```python
from build123d import *

# Parameters (mm, degrees)
F1_DEPTH = 254
F2_R     = 15.875
F3_DEPTH = 12.7


# Not quite as in the source:
# - a pattern or mirror of a feature is missing from the dataset's text; its kind, count and spacing are read off the source's solid


with BuildPart() as f1:
    # F0 (on Front) → F1 (new body)
    with BuildSketch(Plane.XZ):
        Polygon((101.6, 116.5001839399), (0, 0), (203.2, 0), align=None)
    extrude(amount=F1_DEPTH)

    # F2 (on face) → F3 (cut)
    with BuildSketch(Plane(origin=(115.4177397592, 0, 100.6559986685), x_dir=(0, 1, 0), z_dir=(0.7536582036, 0, 0.6572665458))):
        with BuildLine():
            Line((-165.875079947, -18.1667619065), (-171.45, -18.1667619065))
            ThreePointArc((-171.45, -18.1667619065), (-209.55, -56.2667619065), (-171.45, -94.3667619065))
            Line((-171.45, -94.3667619065), (-165.875079947, -94.3667619065))
            ThreePointArc((-165.875079947, -94.3667619065), (-127, -88.270559031), (-88.124920053, -94.3667619065))
            Line((-88.124920053, -94.3667619065), (-82.55, -94.3667619065))
            ThreePointArc((-82.55, -94.3667619065), (-44.45, -56.2667619065), (-82.55, -18.1667619065))
            Line((-82.55, -18.1667619065), (-88.124920053, -18.1667619065))
            ThreePointArc((-88.124920053, -18.1667619065), (-127, -24.262964782), (-165.875079947, -18.1667619065))
        make_face()
        with Locations((-171.45, -56.2667619065)):
            Circle(F2_R, mode=Mode.SUBTRACT)
        with Locations((-82.55, -56.2667619065)):
            Circle(F2_R, mode=Mode.SUBTRACT)
    f3 = extrude(amount=-F3_DEPTH, mode=Mode.SUBTRACT)

    # F3_copies: F3 across plane
    add(f3.mirror(Plane(origin=(101.6, 0, 0), x_dir=(0, 0, -1), z_dir=(-1, 0, 0))), mode=Mode.SUBTRACT)


solid = f1.part
```
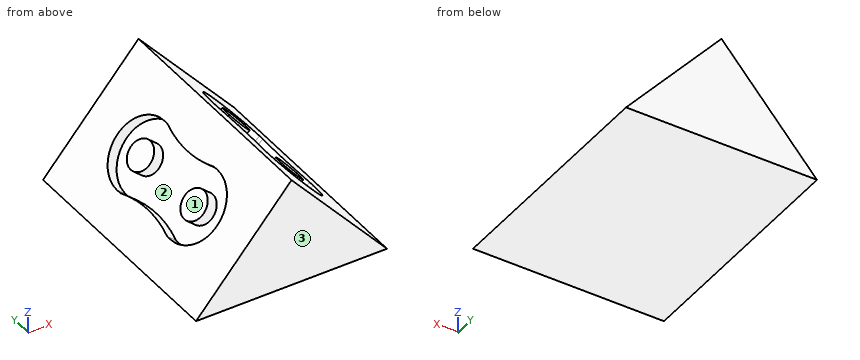
The listing builds one solid part. Answer for the finished solid, in the listing's coordinates (mm). Face numbers are marked on the shaded views. Round coordinates to 2 decimals unless told otherwise and drop trailing zeros. Order: outer loops, then holes, each group sorted by start corner. A loop starts at its lowest first (then second) coordinate and runs counter-clockwise, first axis right, second up. Notation, with made-up numbers: (52.5, 2.5) - (102.5, 2.5) arc R22 ccw to (102.5, 32.5) - close; hole circle Ø5 at (-31, 50.5). An arc over 180 degrees is marked (long way). Put each result on its own line as item: value. Start each with the question number.
(1) Straight lines are drawn through the part: probe 1 along Y at (x, z) = (150.5, 47); probe 2 along Z at (x, y) = (88, -155); probe 3 along X at (y, z) = (-25, 45.5). For each, find the intervals that lie inside material, in ascending order. Write a range as from..to.
(2) Determine the mould class of the marked faces 1, 2 and 3 for opening direction Z: released by +Z, released by -Z, zero draft, split by the parting line, or undercut.
(3) Find section A-A (z = 66.5). State how many separate pieces and enclosed holes the cut face has, plus the area to 3 significant figures.
(4) Find section B-B (y = -132). Give the vertices of the cut face in (x, z), plus the area to 3 significant figures.
(5) Given P1, Ø1, axis at y = -33.5, z = 38, coming from the -X side; P2, Ø4, axis at x = 120, y = -110.5, coming from the +Z side; P3, Ø6, axis at y = -147.5, z = 51, coming from the -X side, each flat-ended and moving along its own axis, determine where each tip first touches the part or whether it passes through.
(6) Find section D-D (x = 182.5). Give the vertices of the cut face in (y, z).
Reply:
1. probe 1: -254..-208.86, -185.58..-157.32, -96.68..-68.42, -45.14..0
1. probe 2: 0..100.91
1. probe 3: 39.68..163.52
2. face 1: released by +Z
2. face 2: undercut
2. face 3: zero draft
3. separate pieces: 5
3. enclosed holes: 0
3. area: 17,300 mm^2
4. outline: (0, 0) - (203.2, 0) - (173.5, 34.06) - (163.93, 25.71) - (121.73, 74.1) - (131.3, 82.44) - (101.6, 116.5) - (71.9, 82.44) - (81.47, 74.1) - (39.27, 25.71) - (29.7, 34.06) - close
4. area: 10,200 mm^2
5. P1: x = 32.7
5. P2: z = 97.7
5. P3: x = 58.71
6. outline: (-254, 0) - (0, 0) - (0, 23.74) - (-254, 23.74) - close
